Source: CAD feature listing. Evaluate the final solid. Frame: model axes, mm. A direction names the side the tool comes from. Round coordinates to 2 decimals unless told otherwise and drop trailing zeros. Loops run counter-clockwise (first coordinate to the right, second up) from the corner with the lowest first, then second, coordinate; pieces in that order, holes last. Notation, with made-up numbers: (-8.5, 79.25) -> (13.5, 79.25) arc R18 cw to (13.5, 103.25) -> close; hole circle Ø10 at (-22.5, 53). An arc over 180 degrees is marked (long way). Return JSON: item names as keys, results as strings. Group by question number.
```python
from build123d import *

# Parameters (mm, degrees)
BASE_EXTRUDE_DEPTH       = 33.274
HOLE1_REACH              = 114.783
SKETCH2_R                = 4.1656
SKETCH3_R                = 9.525
HOLE1A_DEPTH             = 109.593838
HOLE1_PATTERN_COUNT      = 2
HOLE1_PATTERN_PITCH      = 38.1
HOLE1_PATTERN_COUNT_DIR2 = 2
HOLE1_PATTERN_PITCH_DIR2 = 38.1
HOLE2_REACH              = 114.783
SKETCH4_R                = 4.1656
SKETCH5_R                = 9.525
HOLE2A_DEPTH             = 109.593838
HOLE2_PATTERN_COUNT      = 2
HOLE2_PATTERN_PITCH      = 38.1
HOLE2_PATTERN_COUNT_DIR2 = 2
HOLE2_PATTERN_PITCH_DIR2 = 38.1


with BuildPart() as part:
    # Sketch1 → Base Extrude (new body)
    with BuildSketch(Plane(origin=(0, 0, 0), x_dir=(0, 0, -1), z_dir=(1, 0, 0))):
        with BuildLine():
            Line((0, 76.2), (0, 0))
            Line((0, 0), (76.2, 0))
            Line((76.2, 0), (76.2, 3.7084))
            ThreePointArc((76.2, 3.7084), (75.716635, 6.13844), (74.340128, 8.198528))
            Line((74.340128, 8.198528), (8.198528, 74.340128))
            ThreePointArc((8.198528, 74.340128), (6.13844, 75.716635), (3.7084, 76.2))
            Line((3.7084, 76.2), (0, 76.2))
        make_face()
        with BuildLine():
            Line((6.35, 65.98198), (6.35, 6.858))
            ThreePointArc((6.35, 6.858), (6.49879, 6.49879), (6.858, 6.35))
            Line((6.858, 6.35), (65.98198, 6.35))
            ThreePointArc((65.98198, 6.35), (66.45131, 6.663597), (66.34119, 7.21721))
            Line((66.34119, 7.21721), (7.21721, 66.34119))
            ThreePointArc((7.21721, 66.34119), (6.663597, 66.45131), (6.35, 65.98198))
        make_face(mode=Mode.SUBTRACT)
    extrude(amount=-BASE_EXTRUDE_DEPTH)

    # Sketch2 → Hole1 (cut, up to next)
    with BuildSketch(Plane.XZ, mode=Mode.PRIVATE) as hole1_sk1:
        with Locations(Location((-16.637, -19.05, 0), (0, 0, 270))):
            Circle(SKETCH2_R)
    hole1_tool1 = extrude(hole1_sk1.sketch, amount=-HOLE1_REACH, mode=Mode.PRIVATE) & part.part
    hole1 = hole1_tool1.solids().sort_by_distance((-16.637, 0, -19.05))[0]
    add(hole1, mode=Mode.SUBTRACT)

    # Sketch3 → Hole1a (cut, through all)
    with BuildSketch(Plane(origin=(0, 6.35, 0), x_dir=(-1, 0, 0), z_dir=(0, 1, 0))):
        with Locations(Location((16.637, -19.05, 0), (0, 0, 270))):
            Circle(SKETCH3_R)
    hole1a = extrude(amount=HOLE1A_DEPTH, mode=Mode.SUBTRACT)

    # Hole1 Pattern: Hole1, Hole1a 2 × 2
    with Locations(*[(i * HOLE1_PATTERN_PITCH, 0, -j * HOLE1_PATTERN_PITCH_DIR2) for i in range(HOLE1_PATTERN_COUNT) for j in range(HOLE1_PATTERN_COUNT_DIR2) if (i, j) != (0, 0)]):
        add(hole1, mode=Mode.SUBTRACT)
        add(hole1a, mode=Mode.SUBTRACT)

    # Sketch4 → Hole2 (cut, up to next)
    with BuildSketch(Plane.XY, mode=Mode.PRIVATE) as hole2_sk1:
        with Locations((-16.637, 19.05)):
            Circle(SKETCH4_R)
    hole2_tool1 = extrude(hole2_sk1.sketch, amount=-HOLE2_REACH, mode=Mode.PRIVATE) & part.part
    hole2 = hole2_tool1.solids().sort_by_distance((-16.637, 19.05, 0))[0]
    add(hole2, mode=Mode.SUBTRACT)

    # Sketch5 → Hole2a (cut, through all)
    with BuildSketch(Plane(origin=(0, 0, -6.35), x_dir=(-1, 0, 0), z_dir=(0, 0, -1))):
        with Locations((16.637, 19.05)):
            Circle(SKETCH5_R)
    hole2a = extrude(amount=HOLE2A_DEPTH, mode=Mode.SUBTRACT)

    # Hole2 Pattern: Hole2, Hole2a 2 × 2
    with Locations(*[(i * HOLE2_PATTERN_PITCH, j * HOLE2_PATTERN_PITCH_DIR2, 0) for i in range(HOLE2_PATTERN_COUNT) for j in range(HOLE2_PATTERN_COUNT_DIR2) if (i, j) != (0, 0)]):
        add(hole2, mode=Mode.SUBTRACT)
        add(hole2a, mode=Mode.SUBTRACT)


solid = part.part
```
(1) Cut plane C-C (z = -52). Return loops of the section in (x, y) (3 decimals).
(2) Pin query (flat end, axial travel): pin 1 (3 mm diameter, centred on x = -4.5, z = -54, fed in from +Y); pin 2 (17 mm diameter, centred on x = -16.637, z = -19.05, fed in from +Y); pin 3 (7.5 mm diameter, centred on x = -16.637, y = 19.05, fed in from +Z); pin 4 (15 mm diameter, centred on x = -16.637, y = 57.15, fed in from -Z). Return the tip coordinate at first contact, or that it passes through.
(3) Ray query, line 1 (X direction, y = 3.5, z = -57.15); line 2 (Y direction, x = -12, z = -17.5); line 3 (Z direction, x = -24, y = 57.5). Return the intervals inside material, ascending.
(4) Mould query, pull axis Y, two halves, no side actions, for faces 1 (the face through (-16.4, 40.81, -41.73)), 2 (the face through (-16.713, 28.575, -47.433)), 3 (the face through (-12.507, 3.131, -18.508)). Classes: released by +Y, released by -Y, zero draft, split by the parting line, or undercut.
(5) Set-up query: faces 4 (the face through (-16.552, 47.625, -28.846)), 5 (the face through (-18.06, 67.05, -9.63)), 6 (the face through (-16.4, 36.37, -37.19)). Return all of +Z, -Z, +X, -X, +Y, -Y with unobstructed straight access to the full face (end or side cutting, diameter ignored); none if empty.
(6) Cut plane A-A (x = -23). Return loops of the section in (y, z).
(7) Cut plane B-B (z = -32.5). Return loops of the section in (x, y) (3 decimals).
(8) Cut plane D-D (x = -11.5). Return loops of the section in (y, z).
Answers follow:
{
 "1": {"outline": "(-33.274, 0) -> (0, 0) -> (0, 6.35) -> (-33.274, 6.35) -> close; (-33.274, 21.558) -> (-25.826, 21.558) arc R9.525 cw to (-24.65, 24.2) -> (-24.65, 30.539) -> (-33.274, 30.539) -> close; (-8.624, 24.2) arc R9.525 cw to (-7.448, 21.558) -> (0, 21.558) -> (0, 30.539) -> (-8.624, 30.539) -> close"},
 "2": {"pin 1": "y = 30.04", "pin 2": "y = 6.35", "pin 3": "through", "pin 4": "z = -6.35"},
 "3": {"line 1": "-33.27 to -20.8, -12.47 to 0", "line 2": "0 to 6.35", "line 3": "-6.35 to 0"},
 "4": {"face 1": "released by +Y", "face 2": "undercut", "face 3": "zero draft"},
 "5": {"face 4": "-Z", "face 5": "+Y", "face 6": "+X, -X"},
 "6": {"outline": "(0, -76.2) -> (3.71, -76.2) arc R6.35 ccw to (8.2, -74.34) -> (11.96, -70.58) -> (11.96, -64.24) -> (9.32, -64.24) -> (7.22, -66.34) arc R0.51 cw to (6.35, -65.98) -> (6.35, -6.86) arc R0.51 cw to (6.86, -6.35) -> (65.98, -6.35) arc R0.51 cw to (66.34, -7.22) -> (64.24, -9.32) -> (64.24, -11.96) -> (70.58, -11.96) -> (74.34, -8.2) arc R6.35 ccw to (76.2, -3.71) -> (76.2, 0) -> (0, 0) -> close; (26.14, -50.06) -> (32.48, -50.06) -> (50.06, -32.48) -> (50.06, -26.14) -> (47.42, -26.14) -> (26.14, -47.42) -> close"},
 "7": {"outline": "(-33.274, 0) -> (0, 0) -> (0, 6.35) -> (-33.274, 6.35) -> close; (-33.274, 41.058) -> (0, 41.058) -> (0, 50.039) -> (-10.3, 50.039) arc R9.525 cw to (-22.974, 50.039) -> (-33.274, 50.039) -> close"},
 "8": {"outline": "(0, -76.2) -> (3.71, -76.2) arc R6.35 ccw to (8.2, -74.34) -> (11.03, -71.51) -> (11.03, -65.17) -> (8.39, -65.17) -> (7.22, -66.34) arc R0.51 cw to (6.35, -65.98) -> (6.35, -6.86) arc R0.51 cw to (6.86, -6.35) -> (65.98, -6.35) arc R0.51 cw to (66.34, -7.22) -> (65.17, -8.39) -> (65.17, -11.03) -> (71.51, -11.03) -> (74.34, -8.2) arc R6.35 ccw to (76.2, -3.71) -> (76.2, 0) -> (0, 0) -> close; (27.07, -49.13) -> (33.41, -49.13) -> (49.13, -33.41) -> (49.13, -27.07) -> (46.49, -27.07) -> (27.07, -46.49) -> close"}
}
